Read the model definition and answer for the solid it produces. Units are mm, in the model's axes. Face numbers are marked on the shaded views. Give positions to 0.01 mm unless a question says otherwise; leave off trailing zeros. Order: outer loops, then holes, each group sorted by start corner. A loop starts at its lowest first (then second) coordinate and runs counter-clockwise, first axis right, second up. Notation, with made-up numbers: M 87,-39.5 L 138,-39.5 A22 cw 138,-18.5 Z; hole C 24.25,59.25 d1. An arc over 180 degrees is marked long. Write item = value, one per line. Start each with the question number.
Autodesk Inventor part; units mm, degrees
ref_plane "POffset" through (0, 8.3, 0) normal (0, 1, 0) x (-1, 0, 0)
ref_plane "Work Plane3" through (14.2875, 0, 0) normal (1, 0, 0) x (0, 1, 0)
ref_plane "Work Plane4" through (-14.2875, 0, 0) normal (1, 0, 0) x (0, 1, 0)
sketch "Sketch1" plane through (0, 0, 0) normal (0, 0, 1) x (1, 0, 0)
  circle A0 centre (0, 0) radius 14.2875
  circle A1 centre (0, 0) radius 13.0429
  dimension "d0" = 28.575
  dimension "d1" = 26.0858
extrude "Extrusion1" add sketch "Sketch1" along normal blind 81.9912
ref_plane "POffset" through (0, 8.3, 0) normal (0, 1, 0) x (-1, 0, 0)
sketch "Sketch2" plane through (0, 8.3, 0) normal (0, 1, 0) x (-1, 0, 0)
  line L0 (11.6294, 81.9912) -> (11.6294, 0)
  line L1 (11.6294, 0) -> (10.0612, 0)
  line L2 (10.0612, 0) -> (10.0612, 81.9912)
  line L3 (10.0612, 81.9912) -> (11.6294, 81.9912)
  line L4 (-11.6294, 0) -> (-11.6294, 81.9912)
  line L5 (-11.6294, 81.9912) -> (-10.0612, 81.9912)
  line L6 (-10.0612, 81.9912) -> (-10.0612, 0)
  line L7 (-10.0612, 0) -> (-11.6294, 0)
  line L8 (-11.6294, 81.9912) -> (11.6294, 81.9912)
  line L9 (11.6294, 81.9912) -> (11.6294, 48.9912)
  line L10 (11.6294, 48.9912) -> (-11.6294, 48.9912)
  line L11 (-11.6294, 48.9912) -> (-11.6294, 81.9912)
  point P0 (0, 0)
  dimension "d5" = 33
extrude "Extrusion2" cut sketch "Sketch2" along normal through all contours L0 L10 L2 L3 | L2 L10 L6 L8 | L6 L10 L4 L5
ref_plane "Work Plane2" through (0, 14.2875, 0) normal (0, 1, 0) x (-1, 0, 0)
sketch "Sketch3" plane through (0, 14.2875, 0) normal (0, 1, 0) x (-1, 0, 0)
  line L0 (-14.2875, 0) -> (14.2875, 0)
  line L1 (0, -16.3982) -> (0, 98.3894)
  point P0 (0, 0)
  point P1 (0, 2.5)
  dimension "d8" = 2.5
hole "Hole1" at (0, 14.2875, 2.5) direction (0, -1, 0) diameter 1 end up to surface
ref_plane "Work Plane3" through (14.2875, 0, 0) normal (1, 0, 0) x (0, 1, 0)
sketch "Sketch4" plane through (14.2875, 0, 0) normal (1, 0, 0) x (0, 1, 0)
  line L0 (-14.2875, 0) -> (14.2875, 0)
  line L1 (0, -16.3982) -> (0, 98.3894)
  point P0 (0, 0)
  point P1 (0, 2.5)
  dimension "d16" = 2.5
hole "Hole2" at (14.2875, 0, 2.5) direction (-1, 0, 0) diameter 1 end up to surface
ref_plane "Work Plane4" through (-14.2875, 0, 0) normal (1, 0, 0) x (0, 1, 0)
sketch "Sketch5" plane through (-14.2875, 0, 0) normal (1, 0, 0) x (0, 1, 0)
  line L0 (-14.2875, 0) -> (14.2875, 0)
  line L1 (0, -16.3982) -> (0, 98.3894)
  line L2 (1.25, 5) -> (-1.25, 5)
  line L3 (-1.25, 5) -> (-1.25, 0)
  line L4 (-1.25, 0) -> (1.25, 0)
  line L5 (1.25, 0) -> (1.25, 5)
  point P0 (0, 0)
  point P1 (0, 5)
  point P2 (0, 0)
  dimension "d24" = 2.5
  dimension "d25" = 5
extrude "Extrusion3" cut sketch "Sketch5" along normal blind 3
ref_plane "Work Plane5" through (0, -14.2875, 0) normal (0, 1, 0) x (-1, 0, 0)
sketch "Sketch6" plane through (0, -14.2875, 0) normal (0, 1, 0) x (-1, 0, 0)
  line L0 (-13.0429, 81.9912) -> (13.0429, 81.9912)
  line L1 (0, -16.3982) -> (0, 98.3894)
  point P0 (0, 0)
  point P1 (-10.0612, 81.9912)
  point P2 (10.0612, 81.9912)
  point P3 (0, 80.0572)
  dimension "d28" = 1.934
hole "Hole3" at (0, -14.2875, 80.0572) direction (0, 1, 0) diameter 1.1938 end through all
sketch "Sketch7" plane through (0, 14.2875, 0) normal (0, 1, 0) x (-1, 0, 0)
  line L0 (-13.0429, 81.9912) -> (13.0429, 81.9912)
  line L1 (0, -16.3982) -> (0, 98.3894)
  point P0 (0, 0)
  point P1 (-10.0612, 81.9912)
  point P2 (10.0612, 81.9912)
  point P3 (0, 42.9912)
  dimension "d36" = 39
hole "Hole4" at (0, 14.2875, 42.9912) direction (0, -1, 0) diameter 1.7018 depth 3
equation "\"d5\" = length"
equation "\"POffset\" = 8.3"
equation "\"d4\" = POffset"
equation "\"length\" = 33"
properties part number "Main_Tubing_Al"
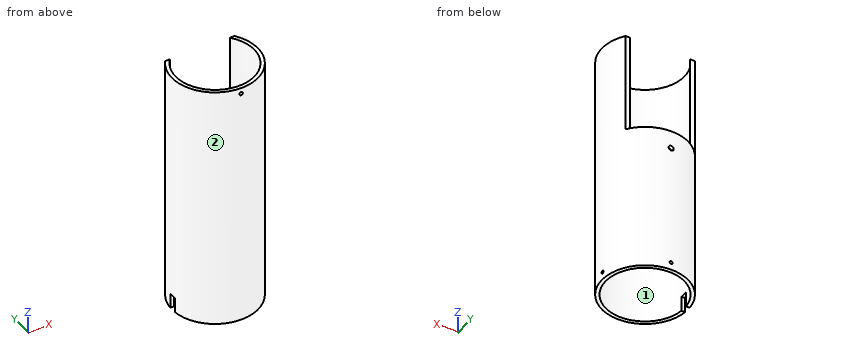
1) Find section B-B on y = -7.75. Determine the outline of the cut face in (x, z).
2) Each of these flat-tipped pins is pushed along its axis until it touches: P1, Ø0.8, axis at x = -10.5, z = 70.5, coming from the +Y side; P2, Ø4, axis at y = 3.5, z = 71, coming from the -X side; P3, Ø2, axis at y = 5, z = 61, coming from the -X side; P4, Ø4, axis at x = -8.5, y = -5, coming from the +Z side. Where does it stop, or does it pass through?
3) Find section C-C on z = 54. Determine the outline of the cut face in (x, y) (1 decimal).
4) Find section A-A on x = 4.25. Determine the outline of the cut face in (y, z), plus the area to 3 significant figures.
5) For a pull along X with two mould halves and no side action, classify the marked faces 1 and 2 as pulls with the +X half, pulls with the -X half, needs draft (parallel to the pull), parting line crosses it, or undercut.
6) Find section D-D on z = 45.5. Determine the outline of the cut face in (x, y) (1 decimal), plus the area to 3 significant figures.
7) Find the intervals of material crossed by probe 1 along Z at (x, y) = (0, 13.55); probe 2 along Y at (x, z) = (0.25, 30); probe 3 along Z at (x, y) = (13.3, 0), in increasing order. Write a range as [from, to].
Numbers:
q1.outline = M -12,0 L -10.49,0 L -10.49,81.99 L -12,81.99 Z; M 10.49,0 L 12,0 L 12,81.99 L 10.49,81.99 Z
q2.P1 = 8.3
q2.P2 = -14.21
q2.P3 = -13.72
q2.P4 = through
q3.outline = M -11.6,8.3 A14.3 ccw long 11.6,8.3 L 10.1,8.3 A13 cw long -10.1,8.3 Z
q4.outline = M -13.64,0 L -12.33,0 L -12.33,81.99 L -13.64,81.99 Z; M 12.33,0 L 13.64,0 L 13.64,48.99 L 12.33,48.99 Z
q4.area = 172 mm2
q5.face_1 = undercut
q5.face_2 = parting line crosses it
q6.outline = C 0,0 d28.6; hole C 0,0 d26.1
q6.area = 107 mm2
q7.probe_1 = [0, 2], [3, 42.14], [43.84, 48.99]
q7.probe_2 = [-14.29, -13.04], [13.04, 14.29]
q7.probe_3 = [0, 2], [3, 81.99]
